Here's how the part is built. I have some questions about the finished solid (model axes, mm). Coordinates: 2 decimals unless noted, no trailing zeros. Write each loop counter-clockwise with the first axis right and the second up, starting at its lowest first coordinate (ties: lowest second). Pieces come first, ordered by that corner, then holes. Notation, with made-up numbers: (16.5, -28) - (53.5, -28) arc R18 cw to (53.5, -6) - close; hole circle Ø4 at (45, -32). An arc over 180 degrees is marked (long way). Answer in a Markdown table with one row per item. Add a question column.
Item 1: I'm going to push a flat-ended pin straight in: pin 1 (2 mm diameter, centred on x = -60.37, z = 0, fed in from -Y). Where does the tip first touch, or does it pass through?
Item 2: If I drill on probe 1 along X at (y, z) = (2.85, -0.25); probe 2 along X at (y, z) = (0.2, -1.25); probe 3 along X at (y, z) = (1.4, 2), over which ranges is the centre line in solid material (lowest first)? Write a range as from..to.
Item 3: Imagine slicing it at A-A (z = 0). Please give me the cut outline in (x, y) (3 decimals), plus the area to 3 significant figures.
Item 4: Imagine slicing it at B-B (y = 1.8). Please give me the cut outline in (x, z) (3 decimals), plus the area to 3 significant figures.
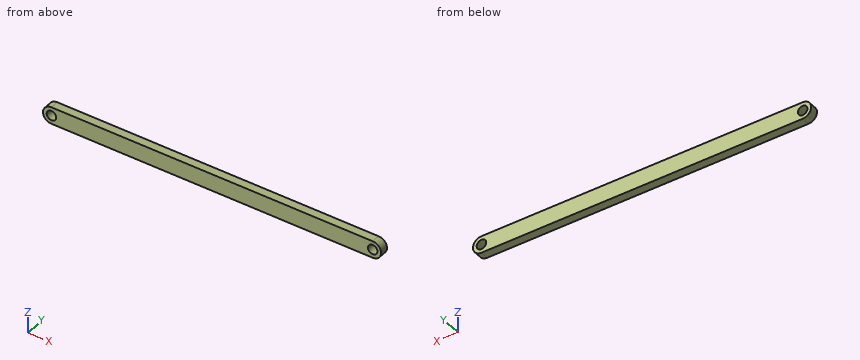
from build123d import *

# Parameters (mm, degrees)
BOSS_EXTRUDE1_DEPTH             = 3.175
F_9_64_0_14063_DIAMETER_HOLE1_D = 3.572002


with BuildPart() as part:
    # Sketch1 → Boss-Extrude1 (new body)
    with BuildSketch(Plane(origin=(0, 0, 0), x_dir=(1, 0, 0), z_dir=(0, 1, 0))):
        with BuildLine():
            Line((60.366783, -3.175), (-60.366783, -3.175))
            ThreePointArc((-60.366783, -3.175), (-63.541783, 0), (-60.366783, 3.175))
            Line((-60.366783, 3.175), (60.366783, 3.175))
            ThreePointArc((60.366783, 3.175), (63.541783, 0), (60.366783, -3.175))
        make_face()
    extrude(amount=BOSS_EXTRUDE1_DEPTH)

    # 9/64 (0.14063) Diameter Hole1 (through all)
    with Locations(Plane(origin=(0, 3.175, 0), x_dir=(1, 0, 0), z_dir=(0, 1, 0))):
        with Locations((60.366783, 0), (-60.366783, 0)):
            Hole(F_9_64_0_14063_DIAMETER_HOLE1_D / 2)


solid = part.part
Here are the results:
| question | item | result |
|---|---|---|
| 1 | pin 1 | passes through |
| 2 | probe 1 | x = -63.53..-62.14, -58.6..58.6, 62.14..63.53 |
| 2 | probe 2 | x = -63.29..-61.64, -59.09..59.09, 61.64..63.29 |
| 2 | probe 3 | x = -62.83..62.83 |
| 3 | outline | (-63.542, 0) - (-62.153, 0) - (-62.153, 3.175) - (-63.542, 3.175) - close; (-58.581, 0) - (58.581, 0) - (58.581, 3.175) - (-58.581, 3.175) - close; (62.153, 0) - (63.542, 0) - (63.542, 3.175) - (62.153, 3.175) - close |
| 3 | area | 381 mm2 |
| 4 | outline | (-60.367, -3.175) - (60.367, -3.175) arc R3.175 ccw to (60.367, 3.175) - (-60.367, 3.175) arc R3.175 ccw to start; hole circle Ø3.572 at (-60.367, 0); hole circle Ø3.572 at (60.367, 0) |
| 4 | area | 778 mm2 |
